```python
from build123d import *

# Parameters (mm, degrees)
SKETCH1_R           = 1.6
BOSS_EXTRUDE1_DEPTH = 2
BOSS_EXTRUDE3_START = 7.4125
BOSS_EXTRUDE3_DEPTH = 7.4125


with BuildPart() as part:
    # Sketch1 → Boss-Extrude1 (new body)
    with BuildSketch(Plane(origin=(0, 0, 0), x_dir=(1, 0, 0), z_dir=(0, 1, 0))):
        with BuildLine():
            Line((-1.5875, 0), (1.5875, 0))
            Line((1.5875, 0), (1.5875, 10))
            Line((1.5875, 10), (13, 10))
            Line((13, 10), (13, -5))
            ThreePointArc((13, -5), (0, -18), (-13, -5))
            Line((-13, -5), (-13, 10))
            Line((-13, 10), (-1.5875, 10))
            Line((-1.5875, 10), (-1.5875, 0))
        make_face()
        with Locations(Location((9.0875, 0, 0), (0, 0, 270))):
            Circle(SKETCH1_R, mode=Mode.SUBTRACT)
        with Locations(Location((-9.0875, 0, 0), (0, 0, 90))):
            Circle(SKETCH1_R, mode=Mode.SUBTRACT)
    boss_extrude1 = extrude(amount=BOSS_EXTRUDE1_DEPTH)

    # Sketch3 → Boss-Extrude3 (add)
    with BuildSketch(Plane.XZ.offset(BOSS_EXTRUDE3_START)):
        with BuildLine():
            Line((4.0875, -10), (1.5875, -10))
            Line((1.5875, -10), (1.5875, 0))
            Line((1.5875, 0), (-1.5875, 0))
            Line((-1.5875, 0), (-1.5875, -10))
            Line((-1.5875, -10), (-4.0875, -10))
            Line((-4.0875, -10), (-4.0875, 5))
            Line((-4.0875, 5), (-13, 5))
            ThreePointArc((-13, 5), (0, 18), (13, 5))
            Line((13, 5), (4.0875, 5))
            Line((4.0875, 5), (4.0875, -10))
        make_face()
    boss_extrude3 = extrude(amount=-BOSS_EXTRUDE3_DEPTH)

    # Mirror11: Boss-Extrude3 across plane
    add(boss_extrude3.mirror(Plane(origin=(0, -7.4125, 0), x_dir=(0, 0, 1), z_dir=(0, -1, 0))))

    # Mirror12: Boss-Extrude1 across plane
    add(boss_extrude1.mirror(Plane(origin=(0, -7.4125, 0), x_dir=(0, 0, 1), z_dir=(0, -1, 0))))


solid = part.part
```
Input: part model. Units: mm. Frame: model coordinates. A direction names the side the tool comes from. Give positions to 0.01 mm unless a question says otherwise; leave off trailing zeros. Write each loop counter-clockwise with the first axis right and the second up, starting at its lowest first coordinate (ties: lowest second). Pieces come first, ordered by that corner, then holes. Notation, with made-up numbers: (46, 41.5) - (98, 41.5) arc R24 cw to (98, 75.5) - close; hole circle Ø11 at (81.5, 88.25). An arc over 180 degrees is marked (long way). Write item = value, one per line. Start each with the question number.
1. Access query for faces 4 (the flat face through (-8, 0, -3)), 5 (the flat face through (0, -7, 0)), 6 (the flat face through (13, 1, -3)), 7 (the flat face through (9, -14.825, -3)), 8 (the flat face through (-13, 1, -2)). Directions: +Z, -Z, +X, -X, +Y, -Y. A direction counts if a zero-diameter tool reaches every point of the face in a straight line with its end or side. Return the directions, or none.
2. Mould query, pull axis X, two halves, no side actions, for faces 1 (the cylindrical face through (-7.526, 0.986, 0.347)), 2 (the flat face through (13, -16, -3)), 3 (the flat face through (-8, -14.825, -3)). Classes: released by +X, released by -X, zero draft, split by the parting line, or undercut.
3. Section query C-C, the plane z = 4.25. Output: boundary loops of the cut face in (x, y) (1 decimal).
4. Section query D-D, the plane y = -7. Output: boundary loops of the cut face in (x, z), then the cut area to 3 significant figures.
5. Section query B-B, the plane y = 0.75. Output: boundary loops of the cut face in (x, z), then the cut area to 3 significant figures.
6. Ray query, L1, parallel to Y at x = 8.25, z = -6.25 (3 decimals); L2, parallel to X at y = -11.75, z = -3.75; L3, parallel to Z at x = 0.25, y = -1.25. Return the intervals inside material, ascending.
7. Section query A-A, the plane z = -1. Count the separate pieces of the cut face and the enclosed holes in it, then the cut area to 3 significant figures.
8. First-contact query: pin 1 Ø10 at (y, z) = (-10.5, 14) entering from -X; pin 2 Ø4 at (y, z) = (-12.5, 6.5) entering from -X; pin 3 Ø3 at (x, y) = (-6.5, -12.5) entering from -Z; pin 4 Ø3 at (y, z) = (-5.5, -5.5) entering from -X. Flat tips, straight axial feed; report the tip coordinate or a pass-through.
Check sheet entries:
q1.face_4 = -Z, -X
q1.face_5 = -Z, +Y, -Y
q1.face_6 = +Z, -Z, +X, +Y, -Y
q1.face_7 = -Z, +X
q1.face_8 = +Z, -Z, -X, +Y, -Y
q2.face_1 = undercut
q2.face_2 = released by +X
q2.face_3 = zero draft
q3.outline = (-13, -16.8) - (13, -16.8) - (13, -14.8) - (4.1, -14.8) - (4.1, 0) - (13, 0) - (13, 2) - (-13, 2) - (-13, 0) - (-4.1, 0) - (-4.1, -14.8) - (-13, -14.8) - close
q4.outline = (-13, 5) - (-4.09, 5) - (-4.09, -10) - (-1.59, -10) - (-1.59, 0) - (1.59, 0) - (1.59, -10) - (4.09, -10) - (4.09, 5) - (13, 5) arc R13 ccw to start
q4.area = 356 mm2
q5.outline = (-13, -10) - (-1.59, -10) - (-1.59, 0) - (1.59, 0) - (1.59, -10) - (13, -10) - (13, 5) arc R13 ccw to (-13, 5) - close; hole circle Ø3.2 at (-9.09, 0); hole circle Ø3.2 at (9.09, 0)
q5.area = 608 mm2
q6.L1 = -16.825 to -14.825, 0 to 2
q6.L2 = -4.09 to -1.59, 1.59 to 4.09
q6.L3 = 0 to 18
q7.separate_pieces = 6
q7.enclosed_holes = 0
q7.area = 145 mm2
q8.pin_1 = -12.37
q8.pin_2 = -13
q8.pin_3 = 5
q8.pin_4 = -4.09
